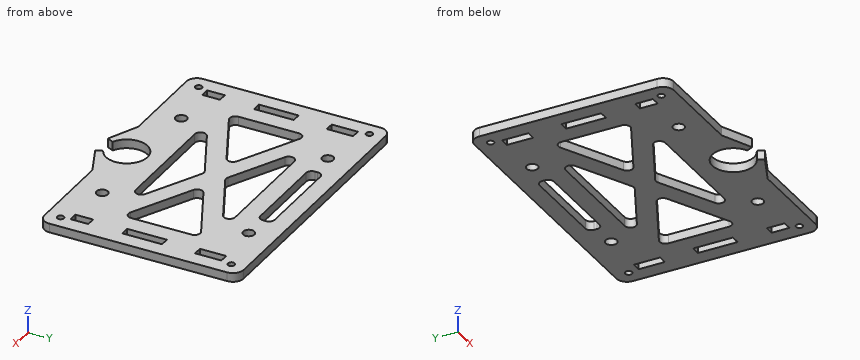
from build123d import *

# Parameters (mm, degrees)
SKETCH1_R           = 0.60325
SKETCH1_W           = 1.5875
SKETCH1_H           = 3.175
SKETCH1_R_2         = 1.016
SKETCH1_H_2         = 7.0993
SKETCH1_H_3         = 4.699
BOSS_EXTRUDE1_DEPTH = 1.5875
SPEED_HOLES_REACH   = 34.529
SKETCH2_W           = 17.145
SKETCH2_H           = 2.54
FILLET1_R           = 1.016


with BuildPart() as part:
    # Sketch1 → Boss-Extrude1 (new body)
    with BuildSketch(Plane.XY):
        with BuildLine():
            ThreePointArc((25.4, 15.875), (24.842038418, 17.222038418), (23.495, 17.78))
            Line((23.495, 17.78), (-23.495, 17.78))
            ThreePointArc((-23.495, 17.78), (-24.842038418, 17.222038418), (-25.4, 15.875))
            Line((-25.4, 15.875), (-25.4, -15.875))
            ThreePointArc((-25.4, -15.875), (-24.842038418, -17.222038418), (-23.495, -17.78))
            Line((-23.495, -17.78), (-7.62, -17.78))
            Line((-7.62, -17.78), (-2.103962754, -20.259962687))
            Line((-2.103962754, -20.259962687), (-1.567237562, -19.108951797))
            ThreePointArc((-1.567237562, -19.108951797), (0, -12.0396), (1.567237562, -19.108951797))
            Line((1.567237562, -19.108951797), (2.103962754, -20.259962687))
            Line((2.103962754, -20.259962687), (7.62, -17.78))
            Line((7.62, -17.78), (23.495, -17.78))
            ThreePointArc((23.495, -17.78), (24.842038418, -17.222038418), (25.4, -15.875))
            Line((25.4, -15.875), (25.4, 15.875))
        make_face()
        with Locations((-22.86, -15.24)):
            Circle(SKETCH1_R, mode=Mode.SUBTRACT)
        with Locations((-21.81225, -12.011129894)):
            Rectangle(SKETCH1_W, SKETCH1_H, mode=Mode.SUBTRACT)
        with Locations((-13.08, -13.08)):
            Circle(SKETCH1_R_2, mode=Mode.SUBTRACT)
        with Locations((13.08, -13.08)):
            Circle(SKETCH1_R_2, mode=Mode.SUBTRACT)
        with Locations((22.86, -15.24)):
            Circle(SKETCH1_R, mode=Mode.SUBTRACT)
        with Locations((21.81225, -12.011129894)):
            Rectangle(SKETCH1_W, SKETCH1_H, mode=Mode.SUBTRACT)
        with Locations((-21.81225, -0.80645)):
            Rectangle(SKETCH1_W, SKETCH1_H_2, mode=Mode.SUBTRACT)
        with Locations((-21.81225, 10.975870106)):
            Rectangle(SKETCH1_W, SKETCH1_H_3, mode=Mode.SUBTRACT)
        with Locations((-22.86, 15.24)):
            Circle(SKETCH1_R, mode=Mode.SUBTRACT)
        with Locations((-13.08, 13.08)):
            Circle(SKETCH1_R_2, mode=Mode.SUBTRACT)
        with Locations((21.81225, -0.80645)):
            Rectangle(SKETCH1_W, SKETCH1_H_2, mode=Mode.SUBTRACT)
        with Locations((21.81225, 10.975870106)):
            Rectangle(SKETCH1_W, SKETCH1_H_3, mode=Mode.SUBTRACT)
        with Locations((13.08, 13.08)):
            Circle(SKETCH1_R_2, mode=Mode.SUBTRACT)
        with Locations((22.86, 15.24)):
            Circle(SKETCH1_R, mode=Mode.SUBTRACT)
    extrude(amount=BOSS_EXTRUDE1_DEPTH)

    # Sketch2 → Speed Holes (cut, up to next)
    with BuildSketch(Plane.XY.offset(1.5875), mode=Mode.PRIVATE) as speed_holes_sk1:
        Polygon((-17.78, -7.044125885), (-3.691748231, 0), (-17.78, 7.044125885), align=None)
    speed_holes_tool1 = extrude(speed_holes_sk1.sketch, amount=-SPEED_HOLES_REACH, mode=Mode.PRIVATE) & part.part
    # Sketch2 → Speed Holes (cut, up to next)
    with BuildSketch(Plane.XY.offset(1.5875), mode=Mode.PRIVATE) as speed_holes_sk2:
        Polygon((-14.088251769, 8.89), (0, 1.845874115), (14.088251769, 8.89), align=None)
    speed_holes_tool2 = extrude(speed_holes_sk2.sketch, amount=-SPEED_HOLES_REACH, mode=Mode.PRIVATE) & part.part
    # Sketch2 → Speed Holes (cut, up to next)
    with BuildSketch(Plane.XY.offset(1.5875), mode=Mode.PRIVATE) as speed_holes_sk3:
        Polygon((3.691748231, 0), (17.78, -7.044125885), (17.78, 7.044125885), align=None)
    speed_holes_tool3 = extrude(speed_holes_sk3.sketch, amount=-SPEED_HOLES_REACH, mode=Mode.PRIVATE) & part.part
    # Sketch2 → Speed Holes (cut, up to next)
    with BuildSketch(Plane.XY.offset(1.5875), mode=Mode.PRIVATE) as speed_holes_sk4:
        Polygon((14.088251769, -8.89), (0, -1.845874115), (-14.088251769, -8.89), align=None)
    speed_holes_tool4 = extrude(speed_holes_sk4.sketch, amount=-SPEED_HOLES_REACH, mode=Mode.PRIVATE) & part.part
    # Sketch2 → Speed Holes (cut, up to next)
    with BuildSketch(Plane.XY.offset(1.5875), mode=Mode.PRIVATE) as speed_holes_sk5:
        with Locations((0, 13.462)):
            Rectangle(SKETCH2_W, SKETCH2_H)
    speed_holes_tool5 = extrude(speed_holes_sk5.sketch, amount=-SPEED_HOLES_REACH, mode=Mode.PRIVATE) & part.part
    add(speed_holes_tool1.solids().sort_by_distance((-13.083916, 0, 1.5875))[0], mode=Mode.SUBTRACT)
    add(speed_holes_tool2.solids().sort_by_distance((0, 6.541958, 1.5875))[0], mode=Mode.SUBTRACT)
    add(speed_holes_tool3.solids().sort_by_distance((13.083916, 0, 1.5875))[0], mode=Mode.SUBTRACT)
    add(speed_holes_tool4.solids().sort_by_distance((0, -6.541958, 1.5875))[0], mode=Mode.SUBTRACT)
    add(speed_holes_tool5.solids().sort_by_distance((0, 13.462, 1.5875))[0], mode=Mode.SUBTRACT)

    # Fillet1
    fillet1_edges = [part.edges().sort_by_distance(p)[0] for p in [
        (-3.691748231, 0, 0.79375),
        (-17.78, -7.044125885, 0.79375),
        (-17.78, 7.044125885, 0.79375),
        (14.088251769, 8.89, 0.79375),
        (0, 1.845874115, 0.79375),
        (-14.088251769, 8.89, 0.79375),
        (17.78, 7.044125885, 0.79375),
        (17.78, -7.044125885, 0.79375),
        (3.691748231, 0, 0.79375),
        (0, -1.845874115, 0.79375),
        (14.088251769, -8.89, 0.79375),
        (-14.088251769, -8.89, 0.79375),
        (-8.5725, 14.732, 0.79375),
        (8.5725, 14.732, 0.79375),
        (8.5725, 12.192, 0.79375),
        (-8.5725, 12.192, 0.79375),
    ]]
    fillet(fillet1_edges, radius=FILLET1_R)


solid = part.part
Source: CAD feature listing. Evaluate the final solid. Frame: model axes, mm. Round coordinates to 2 decimals unless told otherwise and drop trailing zeros. Loops run counter-clockwise (first coordinate to the right, second up) from the corner with the lowest first, then second, coordinate; pieces in that order, holes last. Notation, with made-up numbers: (36, 60.5) - (83, 60.5) arc R18 cw to (83, 64.5) - close; hole circle Ø10 at (-18, -14). An arc over 180 degrees is marked (long way). Write item = value, one per line. Start each with the question number.
(1) Section query D-D, the plane x = 13.08. Output: boundary loops of the cut face in (y, z).
(2) Section query C-C, the plane y = -13.08. Output: boundary loops of the cut face in (x, z), plus the area to 3 significant figures.
(3) Ray query, line 1 along Y through (x, z) = (-22.86, 1.25); line 2 along X through (y, z) = (-2.5, 0.7); line 3 along X through (y, z) = (11.5, 1.2). Return the intervals inside material, ascending. Write a range as from..to.
(4) Section query B-B, the plane x = -15. Output: boundary loops of the cut face in (y, z).
(5) Section query A-A, the plane y = 15.24. Output: boundary loops of the cut face in (x, z).
(6) Pin query (flat end, axial travel): pin 1 (1 mm diameter, centred on x = 22.86, y = 15.24, fed in from +Z); pin 2 (0.5 mm diameter, centred on x = -22, z = 0.5, fed in from -Y); pin 3 (0.5 mm diameter, centred on x = 0.5, z = 0.5, fed in from -Y). Return the tip coordinate at first contact, or that it passes through.
Conclusion:
q1.outline = (-17.78, 0) - (-14.1, 0) - (-14.1, 1.59) - (-17.78, 1.59) - close; (-12.06, 0) - (-4.69, 0) - (-4.69, 1.59) - (-12.06, 1.59) - close; (4.69, 0) - (12.06, 0) - (12.06, 1.59) - (4.69, 1.59) - close; (14.1, 0) - (17.78, 0) - (17.78, 1.59) - (14.1, 1.59) - close
q2.outline = (-25.4, 0) - (-22.61, 0) - (-22.61, 1.59) - (-25.4, 1.59) - close; (-21.02, 0) - (-14.1, 0) - (-14.1, 1.59) - (-21.02, 1.59) - close; (-12.06, 0) - (-2.58, 0) - (-2.58, 1.59) - (-12.06, 1.59) - close; (2.58, 0) - (12.06, 0) - (12.06, 1.59) - (2.58, 1.59) - close; (14.1, 0) - (21.02, 0) - (21.02, 1.59) - (14.1, 1.59) - close; (22.61, 0) - (25.4, 0) - (25.4, 1.59) - (22.61, 1.59) - close
q2.area = 61.0 mm2
q3.line_1 = -17.78..-15.84, -14.64..14.64, 15.84..17.78
q3.line_2 = -25.4..-22.61, -21.02..-17.78, -8.69..-1.31, 1.31..8.69, 17.78..21.02, 22.61..25.4
q3.line_3 = -25.4..-22.61, -21.02..21.02, 22.61..25.4
q4.outline = (-17.78, 0) - (-5.65, 0) - (-5.65, 1.59) - (-17.78, 1.59) - close; (5.65, 0) - (17.78, 0) - (17.78, 1.59) - (5.65, 1.59) - close
q5.outline = (-25.4, 0) - (-23.46, 0) - (-23.46, 1.59) - (-25.4, 1.59) - close; (-22.26, 0) - (22.26, 0) - (22.26, 1.59) - (-22.26, 1.59) - close; (23.46, 0) - (25.4, 0) - (25.4, 1.59) - (23.46, 1.59) - close
q6.pin_1 = through
q6.pin_2 = -17.78
q6.pin_3 = -12.12
